Read the model definition and answer for the solid it produces. Units are mm, in the model's axes. Face numbers are marked on the shaded views. Round coordinates to 2 decimals unless told otherwise and drop trailing zeros. Order: outer loops, then holes, each group sorted by start corner. A loop starts at its lowest first (then second) coordinate and runs counter-clockwise, first axis right, second up. Notation, with made-up numbers: (47.25, 42.25) -> (67.25, 42.25) arc R28 cw to (67.25, 80.25) -> close; hole circle Ø5 at (69.5, 27.25). An arc over 180 degrees is marked (long way). Answer as a JSON object with one key per item and string values. Group by question number.
Item 1: Section C-C, the plane y = 3.75 is taken. Count the separate pieces of the cut face and the enclosed holes in it, plus the area to 3 significant figures.
Item 2: Given P1, Ø0.9, axis at y = 4.5, z = -32.5, coming from the +X side; P2, Ø1, axis at x = 30.5, y = 2, coming from the -Z side; P3, Ø1.3, axis at y = 2, z = 20, coming from the -X side; P4, Ø7, axis at x = -11.5, z = -38.1, coming from the -Y side, each flat-ended and moving along its own axis, determine where each tip first touches the part or whether it passes through.
Item 3: Consider probe 1 along Z at (x, y) = (12.7, 2.75); probe 2 along X at (y, z) = (3.75, -12.7); probe 3 along X at (y, z) = (2.5, 14). Determine where each line is inside the solid, lowest interval first. Write a range as from..to.
Item 4: Section B-B, the plane x = 12.7 is taken. Write down the section's boundary in (y, z).
Item 5: Section D-D, the plane z = -12.7 is taken. Write down the section's boundary in (x, y).
Item 6: Section A-A, the plane z = 6.36 is taken. Write down the section's boundary in (x, y), plus the area to 3 significant figures.
Item 7: The mould has two halves that part along X. Classify the marked faces 1, 2 and 3: pulls with the +X half, pulls with the -X half, needs draft (parallel to the pull), parting line crosses it, or undercut.
from build123d import *

# Parameters (mm, degrees)
BOSS_EXTRUDE1_DEPTH  = 6.35
M5_CLEARANCE_HOLE1_D = 5.5
CUT_EXTRUDE2_DEPTH   = 7.35
FILLET1_R            = 10
SKETCH10_R           = 6.55
CUT_EXTRUDE3_DEPTH   = 7.35
FILLET2_R            = 5


with BuildPart() as part:
    # Sketch1 → Boss-Extrude1 (new body)
    with BuildSketch(Plane(origin=(0, 0, 0), x_dir=(1, 0, 0), z_dir=(0, 1, 0))):
        with BuildLine():
            Line((25.4, -25.4), (-25.4, -25.4))
            Line((-25.4, -25.4), (-25.4, 25.4))
            Line((-25.4, 25.4), (-25.4, 43.35))
            Line((-25.4, 43.35), (1.2, 43.35))
            Line((1.2, 43.35), (1.2, 25.4))
            Line((1.2, 25.4), (25.4, 25.4))
            Line((25.4, 25.4), (89.621209859, 25.4))
            Line((89.621209859, 25.4), (89.621209859, -50.04))
            Line((89.621209859, -50.04), (51.541941751, -50.04))
            ThreePointArc((51.541941751, -50.04), (44.870841587, -48.474895705), (39.591870426, -44.10618968))
            Line((39.591870426, -44.10618968), (25.4, -25.4))
        make_face()
    extrude(amount=BOSS_EXTRUDE1_DEPTH)

    # M5 Clearance Hole1 (through all)
    with Locations(Plane(origin=(0, 6.35, 0), x_dir=(1, 0, 0), z_dir=(0, 1, 0))):
        with Locations((-12.7, 12.7), (12.7, 12.7), (12.7, -12.7), (-12.7, -12.7), (-11.5, 38.1)):
            Hole(M5_CLEARANCE_HOLE1_D / 2)

    # Sketch7 → Cut-Extrude2 (cut, through all)
    with BuildSketch(Plane(origin=(0, 6.35, 0), x_dir=(1, 0, 0), z_dir=(0, 1, 0))):
        with BuildLine():
            Line((53.051764766, -31.105892862), (50.215452987, -32.745892862))
            ThreePointArc((50.215452987, -32.745892862), (49.247834614, -36.366488764), (52.868430515, -37.334107138))
            Line((52.868430515, -37.334107138), (55.704742294, -35.694107138))
            ThreePointArc((55.704742294, -35.694107138), (56.672360668, -32.073511236), (53.051764766, -31.105892862))
        make_face()
        with BuildLine():
            Line((33.75, -19.08), (33.75, -20.72))
            ThreePointArc((33.75, -20.72), (36.4, -23.37), (39.05, -20.72))
            Line((39.05, -20.72), (39.05, -19.08))
            ThreePointArc((39.05, -19.08), (36.4, -16.43), (33.75, -19.08))
        make_face()
    extrude(amount=-CUT_EXTRUDE2_DEPTH, mode=Mode.SUBTRACT)

    # Fillet1
    fillet1_edges = [part.edges().sort_by_distance(p)[0] for p in [
        (-25.4, 3.175, -43.35),
        (1.2, 3.175, -43.35),
        (89.621209859, 3.175, -25.4),
        (89.621209859, 3.175, 50.04),
        (25.4, 3.175, 25.4),
        (-25.4, 3.175, 25.4),
    ]]
    fillet(fillet1_edges, radius=FILLET1_R)

    # Sketch10 → Cut-Extrude3 (cut, through all)
    with BuildSketch(Plane(origin=(0, 6.35, 0), x_dir=(1, 0, 0), z_dir=(0, 1, 0))):
        with Locations((65.621209859, -6.36)):
            Circle(SKETCH10_R)
    extrude(amount=-CUT_EXTRUDE3_DEPTH, mode=Mode.SUBTRACT)

    # Fillet2
    fillet2_edges = [part.edges().sort_by_distance(p)[0] for p in [
        (1.2, 3.175, -25.4),
    ]]
    fillet(fillet2_edges, radius=FILLET2_R)


solid = part.part
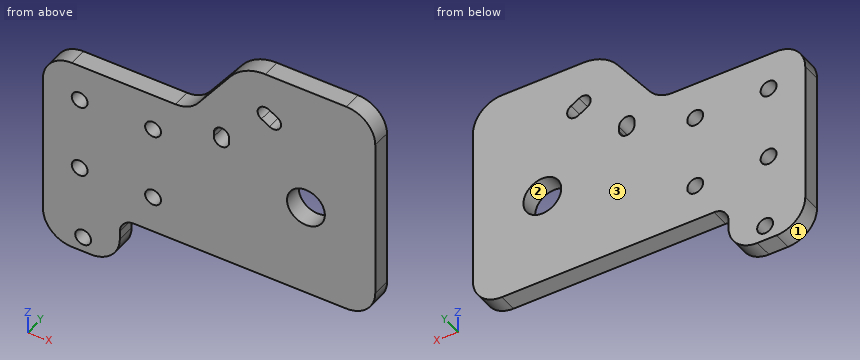
Values found:
{
 "1": {"separate pieces": "1", "enclosed holes": "8", "area": "7,240 mm2"},
 "2": {"P1": "x = 1.2", "P2": "z = -25.4", "P3": "x = -24.59", "P4": "y = 0"},
 "3": {"probe 1": "-25.4..-15.45, -9.95..9.95, 15.45..25.4", "probe 2": "-25.4..-15.45, -9.95..9.95, 15.45..89.62", "probe 3": "-25.4..-15.12, -10.28..10.28, 15.12..89.62"},
 "4": {"outline": "(0, -25.4) -> (6.35, -25.4) -> (6.35, -15.45) -> (0, -15.45) -> close; (0, -9.95) -> (6.35, -9.95) -> (6.35, 9.95) -> (0, 9.95) -> close; (0, 15.45) -> (6.35, 15.45) -> (6.35, 25.4) -> (0, 25.4) -> close"},
 "5": {"outline": "(-25.4, 0) -> (-15.45, 0) -> (-15.45, 6.35) -> (-25.4, 6.35) -> close; (-9.95, 0) -> (9.95, 0) -> (9.95, 6.35) -> (-9.95, 6.35) -> close; (15.45, 0) -> (89.62, 0) -> (89.62, 6.35) -> (15.45, 6.35) -> close"},
 "6": {"outline": "(-25.4, 0) -> (59.07, 0) -> (59.07, 6.35) -> (-25.4, 6.35) -> close; (72.17, 0) -> (89.62, 0) -> (89.62, 6.35) -> (72.17, 6.35) -> close", "area": "647 mm2"},
 "7": {"face 1": "pulls with the -X half", "face 2": "undercut", "face 3": "needs draft"}
}
